Verification items for the finished model (mm, model axes). A direction names the side the tool comes from. Give positions to 0.01 mm unless a question says otherwise; leave off trailing zeros. Order: outer loops, then holes, each group sorted by start corner. A loop starts at its lowest first (then second) coordinate and runs counter-clockwise, first axis right, second up. Notation, with made-up numbers: (42, 39) - (59, 39) arc R20 cw to (59, 53) - close; hole circle Ø2 at (-3.75, 8.25). An arc over 180 degrees is marked (long way). Answer as a JSON object with one key per item and string values.
```python
from build123d import *

# Parameters (mm, degrees)
F0_W     = 210
F0_H     = 140
F0_W_2   = 170
F0_H_2   = 100
F1_DEPTH = 5
F2_W     = 210
F2_H     = 140
F2_W_2   = 206
F2_H_2   = 136
F3_DEPTH = 60
F2_R     = 3.5
F4_DEPTH = 3
F5_D     = 3
F5_DEPTH = 15
F5_TIP   = 0.9012909285
F7_DEPTH = 300


with BuildPart() as f1:
    # F0 (on Top) → F1 (new body)
    with BuildSketch(Plane.XY):
        with Locations((4.9210386318, -0.3193840384)):
            Rectangle(F0_W, F0_H)
        with Locations((4.9210386318, -0.3193840384)):
            Rectangle(F0_W_2, F0_H_2, mode=Mode.SUBTRACT)
    extrude(amount=F1_DEPTH)

    # F2 (on face) → F3 (join)
    with BuildSketch(Plane.XY.offset(5)):
        with Locations((4.9210386318, -0.3193840384)):
            Rectangle(F2_W, F2_H)
        with Locations((4.9210386318, -0.3193840384)):
            Rectangle(F2_W_2, F2_H_2, mode=Mode.SUBTRACT)
    extrude(amount=F3_DEPTH)

    # F2 (on face) → F4 (join)
    with BuildSketch(Plane.XY.offset(5)):
        with Locations((-84.690593183, 49.8957410455)):
            Circle(F2_R)
        with Locations((96.2527468801, 49.8957410455)):
            Circle(F2_R)
        with Locations((-84.690593183, -50.3193840384)):
            Circle(F2_R)
        with Locations((96.2527468801, -50.3193840384)):
            Circle(F2_R)
    extrude(amount=F4_DEPTH)

    # F5 (one way)
    with BuildSketch(Plane(origin=(0, 0, 5), x_dir=(1, 0, 0), z_dir=(0, 0, -1))):
        with Locations((-84.690593183, -49.8957410455), (96.2527468801, -49.8957410455), (-84.690593183, 50.3193840384), (96.2527468801, 50.3193840384)):
            Circle(F5_D / 2)
    extrude(amount=-F5_DEPTH, mode=Mode.SUBTRACT)
    with Locations(Plane(origin=(0, 0, 5), x_dir=(1, 0, 0), z_dir=(0, 0, -1))):
        with Locations((-84.690593183, -49.8957410455), (96.2527468801, -49.8957410455), (-84.690593183, 50.3193840384), (96.2527468801, 50.3193840384)):
            with Locations((0, 0, -(F5_DEPTH + F5_TIP / 2))):  # 118° drill point
                Cone(0, F5_D / 2, F5_TIP, mode=Mode.SUBTRACT)

    # F6 (on face) → F7 (cut)
    with BuildSketch(Plane.YZ.offset(109.9210386318)):
        Polygon((-94.7846397758, 6.4518074505), (80.1731944084, 72.6777166128), (-94.7846397758, 76.6626521945), align=None)
    extrude(amount=-F7_DEPTH, mode=Mode.SUBTRACT)


solid = f1.part
```
(1) Access from +Z, -Z, +X, -X, +Y, -Y to the whole of each face (thin tool, end or side, straight path). Record for faces 1 (the flat face through (3, 69.681, 32)), 2 (the flat face through (4, 49.681, 2)), 3 (the cylindrical face through (98.13, 52.85, 6.48)).
Computed values:
{"face 1": "+Z, -Z, +X, -X, +Y", "face 2": "+Z, -Z", "face 3": "+Z"}
(2) Section check D-D (z = 25). Record the cut outline in (x, y), then the cut area to 3 significant figures.
Computed values:
{"outline": "(-100.08, -45.78) - (-98.08, -45.78) - (-98.08, 67.68) - (107.92, 67.68) - (107.92, -45.78) - (109.92, -45.78) - (109.92, 69.68) - (-100.08, 69.68) - close", "area": "874 mm²"}
(3) Section check C-C (z = 52.5). Record the cut outline in (x, y).
Computed values:
{"outline": "(-100.08, 26.87) - (-98.08, 26.87) - (-98.08, 67.68) - (107.92, 67.68) - (107.92, 26.87) - (109.92, 26.87) - (109.92, 69.68) - (-100.08, 69.68) - close"}
(4) Gauge pin test, flat ends, axial feed: pin 1 Ø10 at (x, y) = (-28, 53) entering from -Z; pin 2 Ø5 at (x, y) = (68, 50) entering from +Z; pin 3 Ø3.5 at (x, y) = (96.5, -50.5) entering from +Z. Record the tip position at first contact, or that the pin passes through.
Computed values:
{"pin 1": "stops at z = 0", "pin 2": "stops at z = 5", "pin 3": "stops at z = 8"}
(5) Material ranges on line 1 along X through (y, z) = (43.5, 44); line 2 along Y through (x, z) = (50.5, 7.5); line 3 along Y through (x, z) = (-31, 37), recorded low to high. Write a range as [from, to].
Computed values:
{"line 1": "x = [-100.08, -98.08], [107.92, 109.92]", "line 2": "y = [-70.32, -68.32], [67.68, 69.68]", "line 3": "y = [67.68, 69.68]"}
(6) Release check for a two-part mould opening along X. For faces 4 (the flat face through (-80.079, -1, 2)), 5 (the flat face through (3, -60, 5)), 6 (the flat face through (109.921, 14, 25)), 7 (the flat face through (3, -70.319, 8)) record: pulls with the +X half, pulls with the -X half, needs draft (parallel to the pull), parting line crosses it, or undercut.
Computed values:
{"face 4": "undercut", "face 5": "undercut", "face 6": "pulls with the +X half", "face 7": "needs draft"}
(7) Section check A-A (x = 36). Record the cut outline in (y, z), then the cut area to 3 significant figures.
Computed values:
{"outline": "(-70.32, 0) - (-50.32, 0) - (-50.32, 5) - (-68.32, 5) - (-68.32, 16.47) - (-70.32, 15.71) - close; (49.68, 0) - (69.68, 0) - (69.68, 65) - (67.68, 65) - (67.68, 5) - (49.68, 5) - close", "area": "342 mm²"}
(8) Section check B-B (y = -1). Record the cut outline in (x, z), then the cut area to 3 significant figures.
Computed values:
{"outline": "(-100.08, 0) - (-80.08, 0) - (-80.08, 5) - (-98.08, 5) - (-98.08, 41.95) - (-100.08, 41.95) - close; (89.92, 0) - (109.92, 0) - (109.92, 41.95) - (107.92, 41.95) - (107.92, 5) - (89.92, 5) - close", "area": "348 mm²"}
